Answer from the drawing. Dimensions are ordinates in mm from the lowest x, y and z of the part. A direction names the side the tool comes from. Coordinates: 2 decimals unless noted, no trailing zeros. Write each loop counter-clockwise with the first axis right and the second up, starting at its lowest first coordinate (ties: lowest second). Pieces come first, ordered by that corner, then holes. Notation, with made-up numbers: (-7.5, -7) - (14.5, -7) arc R12 cw to (14.5, 1) - close; hole circle Ø1 at (-23, -34). An arc over 180 degrees is marked (long way). Answer as a JSON object with one key per item and string values. Group by question number.
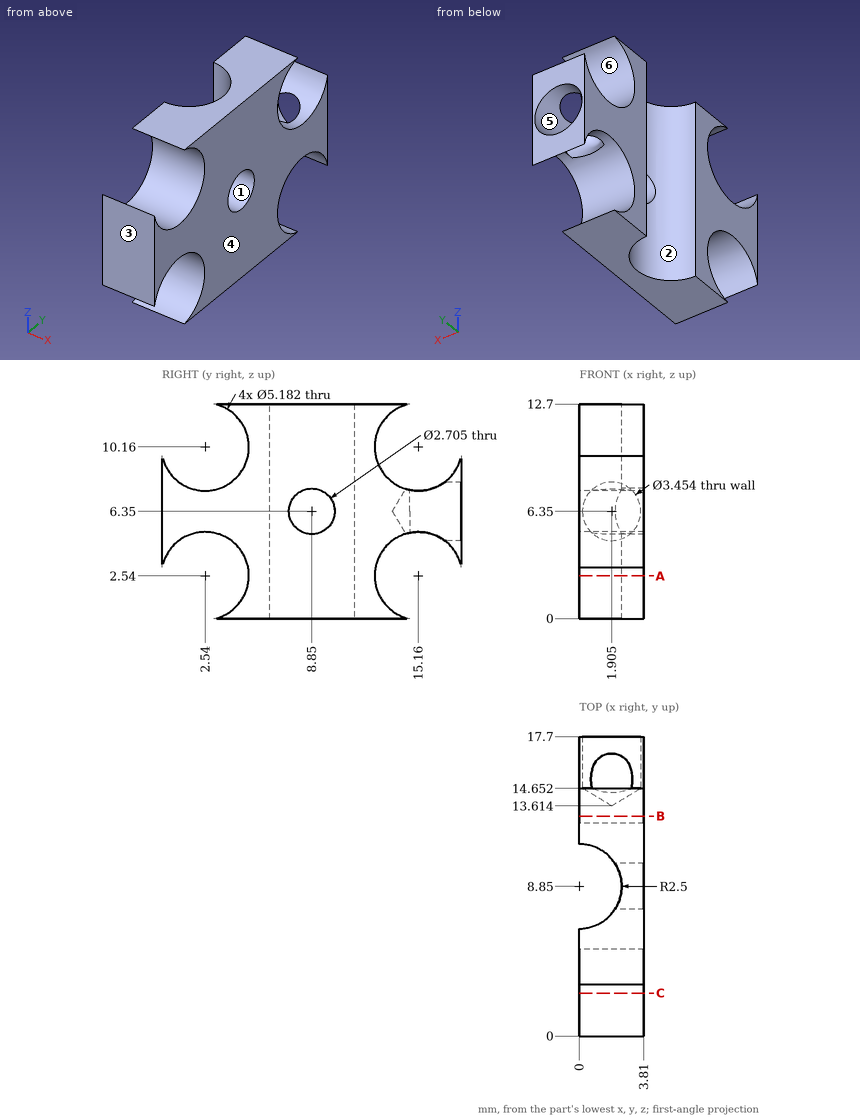
Q1. Section A-A on z = 2.54 is taken. Determine the outline of the cut face in (x, y).
Q2. A tool of negligible diameter and unlimited length cuts with its end or side. For the marked faces 5 and 6, from which of +Z, -Z, +X, -X, +Y, -Y can it reach the whole face along a straight path? Write none if from no direction.
Q3. Consider L1, parallel to Y at x = 0.8, z = 4.75 (1 decimal); L2, parallel to Z at x = 1.1, y = 3.75; L3, parallel to Z at x = 1.05, y = 14 (1 decimal). Determine where each line is inside the solid, lowest interval first. Write a range as from..to.
Q4. For a pull along Y with two mould halves and no side action, classify the marked faces 1, 2, 3 and 4 as +Y half, -Y half, draft (parallel to the pull), parting line (faces both ways), or undercut.
Q5. Section B-B on y = 13 is taken. Determine the outline of the cut face in (x, z), plus the area to 3 significant figures.
Q6. Section C-C on y = 2.54 is taken. Determine the outline of the cut face in (x, z).
Numbers:
{
 "1": {"outline": "(0, 5.13) - (3.81, 5.13) - (3.81, 12.57) - (0, 12.57) - (0, 11.35) arc R2.5 cw to (0, 6.35) - close"},
 "2": {"face 5": "+Y", "face 6": "+X, -X"},
 "3": {"L1": "y = 0..1.2, 3.9..6.5, 11.2..13.8, 16.5..17.7", "L2": "z = 0..0.25, 4.83..7.87, 12.45..12.7", "L3": "z = 0..0.2, 4.9..7.8, 12.5..12.7"},
 "4": {"face 1": "undercut", "face 2": "undercut", "face 3": "-Y half", "face 4": "draft"},
 "5": {"outline": "(0, 0) - (3.81, 0) - (3.81, 1.11) - (0, 1.11) - close; (0, 3.97) - (3.81, 3.97) - (3.81, 8.73) - (0, 8.73) - close; (0, 11.59) - (3.81, 11.59) - (3.81, 12.7) - (0, 12.7) - close", "area": "26.6 mm²"},
 "6": {"outline": "(0, 5.13) - (3.81, 5.13) - (3.81, 7.57) - (0, 7.57) - close"}
}
